Source: CAD feature listing. Evaluate the final solid. Frame: model axes, mm. A direction names the side the tool comes from. Give positions to 0.01 mm unless a question says otherwise; leave off trailing zeros. Write each loop counter-clockwise with the first axis right and the second up, starting at its lowest first coordinate (ties: lowest second). Pieces come first, ordered by that corner, then holes. Notation, with made-up numbers: (-10, 3.25) -> (1, 3.25) arc R14 ccw to (1, 10.25) -> close; hole circle Ø11 at (-31, 21). An arc over 180 degrees is marked (long way). Write item = value, one per line.
from build123d import *

# Parameters (mm, degrees)
SKETCH3_W           = 16.588644014
SKETCH3_H           = 65
SKETCH3_R           = 2.1
SKETCH3_W_2         = 60
SKETCH3_H_2         = 15
BOSS_EXTRUDE1_DEPTH = 4
CUT_EXTRUDE1_DEPTH  = 3
CUT_EXTRUDE2_DEPTH  = 3


with BuildPart() as part:
    # Sketch3 → Boss-Extrude1 (new body)
    with BuildSketch(Plane(origin=(0, 0, 0), x_dir=(1, 0, 0), z_dir=(0, 1, 0))):
        with Locations((39.448385229, -314.860414745)):
            Rectangle(SKETCH3_W, SKETCH3_H)
        with Locations((39.448385229, -332.360414745)):
            Circle(SKETCH3_R, mode=Mode.SUBTRACT)
        with Locations((39.448385229, -297.360414745)):
            Circle(SKETCH3_R, mode=Mode.SUBTRACT)
        with Locations((39.448385229, -274.860414745)):
            Rectangle(SKETCH3_W_2, SKETCH3_H_2)
        with Locations((59.448385229, -274.860414745)):
            Circle(SKETCH3_R, mode=Mode.SUBTRACT)
        with Locations((19.448385229, -274.860414745)):
            Circle(SKETCH3_R, mode=Mode.SUBTRACT)
    extrude(amount=BOSS_EXTRUDE1_DEPTH)

    # Sketch4 → Cut-Extrude1 (cut)
    with BuildSketch(Plane(origin=(0, 4, 0), x_dir=(1, 0, 0), z_dir=(0, 1, 0))):
        Polygon((15.848385229, -276.960414745), (15.848385229, -272.760414745), (19.448385229, -270.760414745), (23.048385229, -272.760414745), (23.048385229, -276.960414745), (19.448385229, -278.960414745), align=None)
        Polygon((55.848385229, -276.960414745), (55.848385229, -272.760414745), (59.448385229, -270.760414745), (63.048385229, -272.760414745), (63.048385229, -276.960414745), (59.448385229, -278.960414745), align=None)
    extrude(amount=-CUT_EXTRUDE1_DEPTH, mode=Mode.SUBTRACT)

    # Sketch5 → Cut-Extrude2 (cut)
    with BuildSketch(Plane(origin=(0, 4, 0), x_dir=(1, 0, 0), z_dir=(0, 1, 0))):
        Polygon((39.448385229, -301.460414745), (43.048385229, -299.460414745), (43.048385229, -295.260414745), (39.448385229, -293.260414745), (35.848385229, -295.260414745), (35.848385229, -299.460414745), align=None)
        Polygon((39.448385229, -328.260414745), (35.848385229, -330.260414745), (35.848385229, -334.460414745), (39.448385229, -336.460414745), (43.048385229, -334.460414745), (43.048385229, -330.260414745), align=None)
    extrude(amount=-CUT_EXTRUDE2_DEPTH, mode=Mode.SUBTRACT)


solid = part.part
1) Draft query along X for faces 1 (the flat face through (47.743, 2, 315)), 2 (the flat face through (17.623, 2.521, 271.774)), 3 (the flat face through (46, 4, 298)), 4 (the flat face through (37.67, 2.52, 294.25)). Return one class per face: pulls with the +X half, pulls with the -X half, needs draft (parallel to the pull), parting line crosses it, or undercut.
Computed:
face_1 = pulls with the +X half
face_2 = undercut
face_3 = needs draft
face_4 = undercut
2) Access query for faces 5 (the flat face through (41.274, 2.521, 329.274)), 6 (the flat face through (46, 0, 298)). Directions: +Z, -Z, +X, -X, +Y, -Y. A direction counts if a zero-diameter tool reaches every point of the face in a straight line with its end or side. Return the directions, or none.
Computed:
face_5 = +Y
face_6 = +Z, -Z, +X, -X, -Y
3) Contact query for flat-ended pins moving along their axis: pin 1 (8 mm diameter, centred on x = 38.5, z = 330.5, fed in from +Y); pin 2 (6.5 mm diameter, centred on x = 19.45, z = 274.86, fed in from +Y); pin 3 (0.9 mm diameter, centred on y = 2.5, z = 333, fed in from +X); pin 4 (0.9 mm diameter, centred on y = 3, z = 332.5, fed in from -X). Output: stop coordinate, or through.
Computed:
pin_1 = 4
pin_2 = 1
pin_3 = 47.74
pin_4 = 31.15
4) Cut plane B-B (x = 40.5). Return the cut outline in (y, z), then the cut area to 3 significant figures.
Computed:
outline = (0, 267.36) -> (4, 267.36) -> (4, 293.84) -> (1, 293.84) -> (1, 295.54) -> (0, 295.54) -> close; (0, 299.18) -> (1, 299.18) -> (1, 300.88) -> (4, 300.88) -> (4, 328.84) -> (1, 328.84) -> (1, 330.54) -> (0, 330.54) -> close; (0, 334.18) -> (1, 334.18) -> (1, 335.88) -> (4, 335.88) -> (4, 347.36) -> (0, 347.36) -> close
area = 271 mm²
5) Cut plane D-D (z = 316.5). Return the cut outline in (x, y).
Computed:
outline = (31.15, 0) -> (47.74, 0) -> (47.74, 4) -> (31.15, 4) -> close
6) Cut plane C-C (z = 333.5). Return the cut outline in (x, y), then the cut area to 3 significant figures.
Computed:
outline = (31.15, 0) -> (37.68, 0) -> (37.68, 1) -> (35.85, 1) -> (35.85, 4) -> (31.15, 4) -> close; (41.21, 0) -> (47.74, 0) -> (47.74, 4) -> (43.05, 4) -> (43.05, 1) -> (41.21, 1) -> close
area = 41.2 mm²
7) Cut plane A-A (y = 3.25). State how many separate pieces and enclosed holes the cut face has, then the cut area to 3 significant figures.
Computed:
separate_pieces = 1
enclosed_holes = 4
area = 1,800 mm²
8) Material intervals for L1, parallel to X at y = 3.8, z = 299; L2, parallel to Z at x = 38, y = 2; L3, parallel to X at y = 2.8, z = 278.5, sorted ascending.
Computed:
L1 = 31.15 to 35.85, 43.05 to 47.74
L2 = 267.36 to 294.07, 300.66 to 329.07, 335.66 to 347.36
L3 = 9.45 to 18.62, 20.28 to 58.62, 60.28 to 69.45
